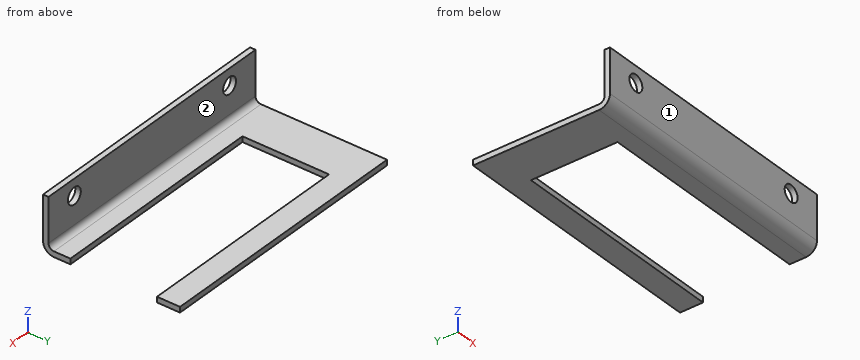
```python
from build123d import *

# Parameters (mm, degrees)
BOSS_EXTRUDE1_DEPTH    = 60.96
CONVERT_SOLID1_DEPTH   = 60.96
CONVERT_SOLID1_2_DEPTH = 60.96
SKETCH6_W              = 40.386
SKETCH6_H              = 20.066
CUT_EXTRUDE1_DEPTH     = 70.67660296
SKETCH8_R              = 1.89865
CUT_EXTRUDE2_DEPTH     = 70.328507845
SKETCH11_W             = 18.1335173
SKETCH11_H             = 20.066
CUT_EXTRUDE5_DEPTH     = 70.67660296


# Read off the part's stored shape, not the designer's step: Convert-Solid1
with BuildPart() as part:
    # Sketch1 → Boss-Extrude1 (new body)
    with BuildSketch(Plane(origin=(0, 0, 0), x_dir=(0, 0, -1), z_dir=(1, 0, 0))):
        Polygon((0, 0), (12.7, 0), (12.7, 31.75), (11.43, 31.75), (11.43, 1.27), (0, 1.27), align=None)
    extrude(amount=BOSS_EXTRUDE1_DEPTH)

    # Convert-Solid1 outline → Convert-Solid1 (cut)
    with BuildSketch(Plane.YZ):
        with BuildLine():
            ThreePointArc((2.54, -12.7), (0.743948776, -11.956051224), (0, -10.16))
            Line((0, -10.16), (0, -12.7))
            Line((0, -12.7), (2.54, -12.7))
        make_face()
    extrude(amount=CONVERT_SOLID1_DEPTH, mode=Mode.SUBTRACT)

    # Convert-Solid1 2 outline → Convert-Solid1 2 (add)
    with BuildSketch(Plane.YZ):
        with BuildLine():
            ThreePointArc((2.54, -11.43), (1.641974388, -11.058025612), (1.27, -10.16))
            Line((1.27, -10.16), (1.27, -11.43))
            Line((1.27, -11.43), (2.54, -11.43))
        make_face()
    extrude(amount=CONVERT_SOLID1_2_DEPTH)

    # Sketch6 → Cut-Extrude1 (cut, through all)
    with BuildSketch(Plane.XY.offset(-11.43)):
        with Locations((30.48, 16.383)):
            Rectangle(SKETCH6_W, SKETCH6_H)
    extrude(amount=-CUT_EXTRUDE1_DEPTH, mode=Mode.SUBTRACT)

    # Sketch8 → Cut-Extrude2 (cut, through all)
    with BuildSketch(Plane(origin=(0, 1.27, 0), x_dir=(1, 0, 0), z_dir=(0, 1, 0))):
        with Locations(Location((7.62, 3.81, 0), (0, 0, 270))):
            Circle(SKETCH8_R)
        with Locations(Location((53.34, 3.81, 0), (0, 0, 270))):
            Circle(SKETCH8_R)
    extrude(amount=-CUT_EXTRUDE2_DEPTH, mode=Mode.SUBTRACT)

    # Sketch11 → Cut-Extrude5 (cut, through all)
    with BuildSketch(Plane.XY.offset(-11.43)):
        with Locations((59.73975865, 16.383)):
            Rectangle(SKETCH11_W, SKETCH11_H)
    extrude(amount=-CUT_EXTRUDE5_DEPTH, mode=Mode.SUBTRACT)


solid = part.part
```
The model under review builds one solid part; all positions refer to its coordinate system, in mm. Face numbers are marked on the shaded views. A direction names the side the tool comes from. Give positions to 0.01 mm unless a question says otherwise; leave off trailing zeros. Loops run counter-clockwise (first coordinate to the right, second up) from the corner with the lowest first, then second, coordinate; pieces in that order, holes last. Notation, with made-up numbers: (67, 66) - (87, 66) arc R19 cw to (87, 99) - close; hole circle Ø8 at (89, 80.25). An arc over 180 degrees is marked (long way). Answer as a JSON object with one key per item and string values.
Q1. To check wall thickness, follow line 1 along X through (y, z) = (0.3, -3.81); line 2 along Y through (x, z) = (19.5, -6.75); line 3 along Y through (x, z) = (56, -11.5). State the ranges of each line that lie inside material, in increasing order.
Worked out:
{"line 1": "x = 0 to 5.72, 9.52 to 51.44, 55.24 to 60.96", "line 2": "y = 0 to 1.27", "line 3": "y = 0.38 to 6.35, 26.42 to 31.75"}
Q2. Add section D-D on y = 10. State the section outline as (x, z) points, plus the area to 3 significant figures.
Worked out:
{"outline": "(0, -12.7) - (10.29, -12.7) - (10.29, -11.43) - (0, -11.43) - close", "area": "13.1 mm^2"}
Q3. Insertion check: pin 1 (1 mm diameter, centred on y = 13.5, z = -12, fed in from +X); pin 2 (2 mm diameter, centred on x = 16, z = -3, fed in from +Y); pin 3 (8 mm diameter, centred on x = 37.5, y = 6.5, fed in from -Z); pin 4 (9 mm diameter, centred on x = 38.5, y = 20, fed in from +Z). Each pin has a flat end and moves straight along its axis. Give the tip position at first contact, or say it passes through.
Worked out:
{"pin 1": "stops at x = 10.29", "pin 2": "stops at y = 1.27", "pin 3": "stops at z = -12.7", "pin 4": "passes through"}
Q4. Add section C-C on x = 53.34. State the section outline as (y, z) points, plus the area to 3 significant figures.
Worked out:
{"outline": "(0, -10.16) arc R2.54 ccw to (2.54, -12.7) - (6.35, -12.7) - (6.35, -11.43) - (2.54, -11.43) arc R1.27 cw to (1.27, -10.16) - (1.27, -5.71) - (0, -5.71) - close; (0, -1.91) - (1.27, -1.91) - (1.27, 0) - (0, 0) - close; (26.42, -12.7) - (31.75, -12.7) - (31.75, -11.43) - (26.42, -11.43) - close", "area": "23.5 mm^2"}
Q5. Add section B-B on z = -3.81. State the section outline as (x, y) points.
Worked out:
{"outline": "(0, 0) - (5.72, 0) - (5.72, 1.27) - (0, 1.27) - close; (9.52, 0) - (51.44, 0) - (51.44, 1.27) - (9.52, 1.27) - close; (55.24, 0) - (60.96, 0) - (60.96, 1.27) - (55.24, 1.27) - close"}
Q6. For the marked faces 1 and 2, list the 3-axis set-ups (+Z, -Z, +X, -X, +Y, -Y) from which the entire face can be reached by the end or side of a thin tool; tool diameter is ignored.
Worked out:
{"face 1": "+Z, -Z, +X, -X, -Y", "face 2": "+Z, +X, -X, +Y"}
Q7. Add section A-A on x = 33. State the section outline as (y, z) points.
Worked out:
{"outline": "(0, -10.16) arc R2.54 ccw to (2.54, -12.7) - (6.35, -12.7) - (6.35, -11.43) - (2.54, -11.43) arc R1.27 cw to (1.27, -10.16) - (1.27, 0) - (0, 0) - close; (26.42, -12.7) - (31.75, -12.7) - (31.75, -11.43) - (26.42, -11.43) - close"}
